Check sheet for the modelled part. Datum: model origin and axes. Units: mm. Face numbers are marked on the shaded views. A direction names the side the tool comes from. Round coordinates to 2 decimals unless told otherwise and drop trailing zeros. Loops run counter-clockwise (first coordinate to the right, second up) from the corner with the lowest first, then second, coordinate; pieces in that order, holes last. Notation, with made-up numbers: M 53.5,-17.5 L 62.5,-17.5 A27 cw 62.5,9.5 Z; hole C 5.25,36.25 d11. An arc over 180 degrees is marked long. One line per question, with ' | ' between items. Start each with the question number.
(1) Draft check along Z on the marked faces 3, 4, 5 and 6. Enter one of: +Z half, -Z half, draft (parallel to the pull), parting line (faces both ways), or undercut.
(2) Section check A-A (y = 3). Record the boundary of the cut face in (x, z).
(3) Thickness scan on probe 1 along Z at (x, y) = (5.25, 31); probe 2 along Y at (x, z) = (3.5, 18.5); probe 3 along X at (y, z) = (0.45, 21). Record the ranges inside material, lowest first. Write a range as [from, to].
(4) Section check D-D (x = 15.5). Record the boundary of the cut face in (y, z).
(5) Section check B-B (x = 24). Record the boundary of the cut face in (y, z).
(6) Go/stop test with a flat-tipped pin: P1, Ø7, axis at y = 22, z = 21, coming from the -X side. Record where the tip stops, or that it passes through.
(7) Tool access check on the marked faces 1 and 2. Record the directions out of +Z, -Z, +X, -X, +Y, -Y that give a thin tool (end or side, any length) a straight path to the whole face; none if there is none.
(8) Section check C-C (z = 10). Record the boundary of the cut face in (x, y), and give its area (3 significant figures).
```python
from build123d import *

# Parameters (mm, degrees)
EXTRUDE_1_DEPTH     = 30
EXTRUDE_2_DEPTH     = 3
CUT_EXTRUDE_1_DEPTH = 3
CUT_EXTRUDE_START   = -17
SKETCH_4_R          = 1.65
CUT_EXTRUDE_2_DEPTH = 76
CUT_EXTRUDE_3_DEPTH = 3
FILLET_1_R          = 5


with BuildPart() as part:
    # Эскиз1 → Бобышка-Вытянуть1 (new body)
    with BuildSketch(Plane.XY):
        Polygon((0, 0), (30, 0), (30, 35), (0, 35), (0, 30), (25, 30), (25, 5), (0, 5), align=None)
    extrude(amount=EXTRUDE_1_DEPTH)

    # Эскиз2 → Бобышка-Вытянуть2 (add)
    with BuildSketch(Plane.XY.offset(30)):
        with BuildLine():
            Line((12.5, 30), (25, 30))
            Line((25, 30), (25, 5))
            Line((25, 5), (12.5, 5))
            ThreePointArc((12.5, 5), (21.929285786, 17.5), (12.5, 30))
        make_face()
    extrude_2 = extrude(amount=-EXTRUDE_2_DEPTH)

    # Зеркальное отражение1: Бобышка-Вытянуть2 across plane
    add(extrude_2.mirror(Plane.XY.offset(15)))

    # Эскиз3 → Вырез-Вытянуть1 (cut)
    with BuildSketch(Plane(origin=(0, 5, 0), x_dir=(1, 0, 0), z_dir=(0, 1, 0))):
        Polygon((4.517949192, -24), (2.785898385, -21), (4.517949192, -18), (7.982050808, -18), (9.714101615, -21), (7.982050808, -24), align=None)
        Polygon((2.785898385, -9), (4.517949192, -12), (7.982050808, -12), (9.714101615, -9), (7.982050808, -6), (4.517949192, -6), align=None)
    extrude(amount=-CUT_EXTRUDE_1_DEPTH, mode=Mode.SUBTRACT)

    # Эскиз4 → Вырез-Вытянуть2 (cut)
    with BuildSketch(Plane(origin=(0, 2, 0), x_dir=(1, 0, 0), z_dir=(0, 1, 0)).offset(CUT_EXTRUDE_START)):
        with Locations(Location((6.25, -21, 0), (0, 0, 90))):
            Circle(SKETCH_4_R)
    cut_extrude_2 = extrude(amount=CUT_EXTRUDE_2_DEPTH, mode=Mode.SUBTRACT)

    # Зеркальное отражение2: Вырез-Вытянуть2 across plane
    add(cut_extrude_2.mirror(Plane.XY.offset(15)), mode=Mode.SUBTRACT)

    # Эскиз5 → Вырез-Вытянуть3 (cut)
    with BuildSketch(Plane.XZ.offset(-30)):
        Polygon((9.714101615, 21), (7.982050808, 24), (4.517949192, 24), (2.785898385, 21), (4.517949192, 18), (7.982050808, 18), align=None)
    cut_extrude_3 = extrude(amount=-CUT_EXTRUDE_3_DEPTH, mode=Mode.SUBTRACT)

    # Зеркальное отражение3: Вырез-Вытянуть3 across plane
    add(cut_extrude_3.mirror(Plane.XY.offset(15)), mode=Mode.SUBTRACT)

    # Скругление1
    fillet_1_edges = [part.edges().sort_by_distance(p)[0] for p in [
        (0, 2.5, 0),
        (0, 32.5, 30),
        (0, 2.5, 30),
        (0, 32.5, 0),
    ]]
    fillet(fillet_1_edges, radius=FILLET_1_R)


solid = part.part
```
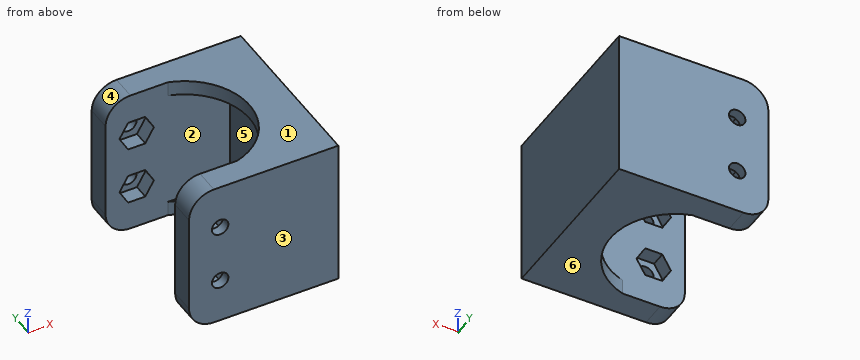
The answers:
1) face 3: draft | face 4: +Z half | face 5: undercut | face 6: -Z half
2) outline: M 0,5 A5 ccw 5,0 L 30,0 L 30,30 L 5,30 A5 ccw 0,25 Z; hole M 2.79,9 L 4.52,6 L 7.98,6 L 9.71,9 L 7.98,12 L 4.52,12 Z; hole M 2.79,21 L 4.52,18 L 7.98,18 L 9.71,21 L 7.98,24 L 4.52,24 Z
3) probe 1: [0, 6], [12, 18], [24, 30] | probe 2: [0, 5], [30, 35] | probe 3: [0, 4.6], [7.9, 30]
4) outline: M 0,0 L 6.28,0 L 6.28,3 L 5,3 L 5,27 L 6.28,27 L 6.28,30 L 0,30 Z; M 28.72,0 L 35,0 L 35,30 L 28.72,30 L 28.72,27 L 30,27 L 30,3 L 28.72,3 Z
5) outline: M 0,0 L 35,0 L 35,30 L 0,30 Z; hole M 5,3 L 30,3 L 30,27 L 5,27 Z
6) P1: x = 25
7) face 1: +Z, +X, -X, +Y, -Y | face 2: -X
8) outline: M 0,0 L 4.94,0 L 4.94,2 L 3.36,2 L 3.36,5 L 0,5 Z; M 0,30 L 3.36,30 L 3.36,33 L 4.94,33 L 4.94,35 L 0,35 Z; M 7.56,0 L 30,0 L 30,35 L 7.56,35 L 7.56,33 L 9.14,33 L 9.14,30 L 25,30 L 25,5 L 9.14,5 L 9.14,2 L 7.56,2 Z | area: 380 mm²
